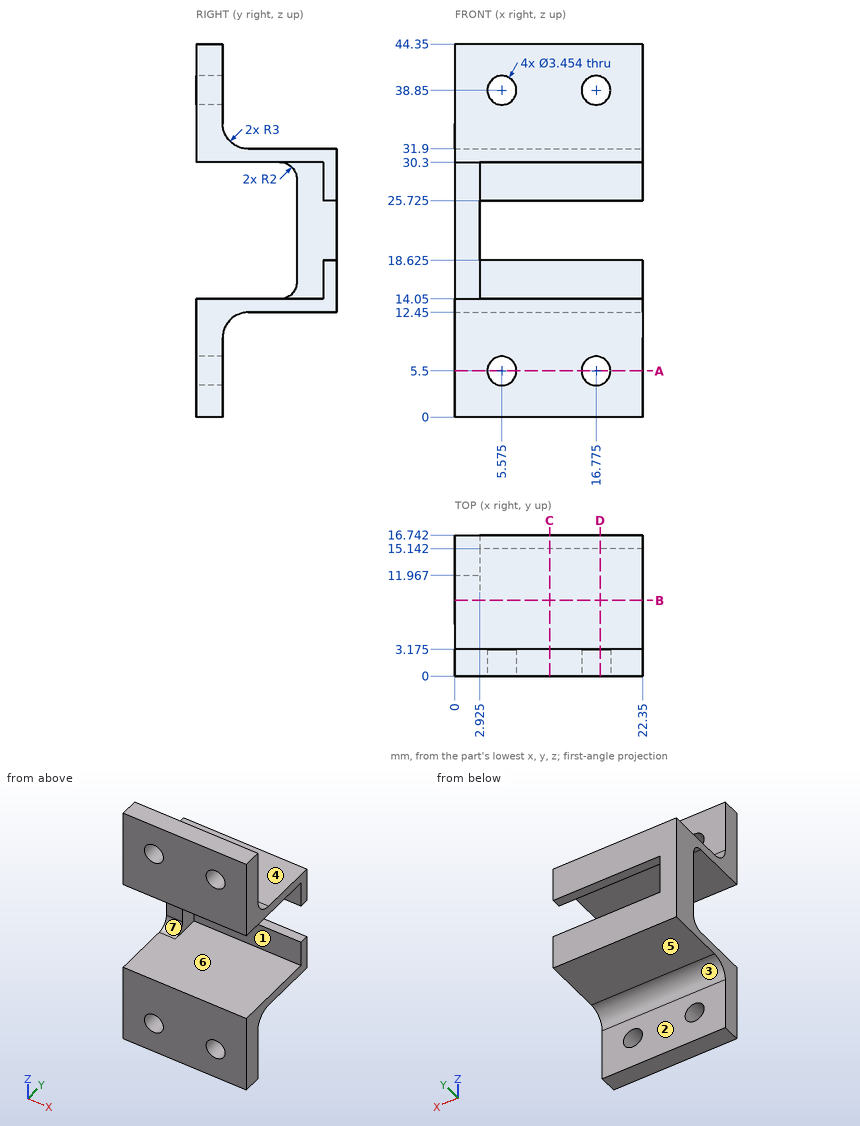
Part print with two shaded views. Sizes in mm from the minimum x, y, z corner. A direction names the side the tool comes from. Give positions to 0.01 mm unless a question says otherwise; leave off trailing zeros. Order: outer loops, then holes, each group sorted by start corner. A loop starts at its lowest first (then second) coordinate and runs counter-clockwise, first axis right, second up.
(1) Saw through at B-B, the plane y = 9. Give the cut face in (x, z), then the cut area to 3 significant figures.
(2) Saw through at C-C, the plane x = 11.25. Give the cut face in (y, z) (3 decimals), then the cut area to 3 significant figures.
(3) Saw through at D-D, the plane x = 17.25. Give the cut face in (y, z) (3 decimals).
(4) Tool access for the marked faces 5, 6 and 7: list every direction of +Z, -Z, +X, -X, +Y, -Y with a clear straight run to the whole face (end or side of a thin tool).
(5) Mould opens along Z. For the marked faces 1, 2, 3 and 4 say: released by +Z, released by -Z, zero draft, split by the parting line, or undercut.
(6) Saw through at A-A, the plane z = 5.5. Give the cut face in (x, y) (3 decimals).
(7) Drill centre lines: L1, parallel to X at y = 1.8, z = 5.5; L2, parallel to Z at x = 14, y = 14; L3, parallel to Z at x = 7.75, y = 2. Where is each one in solid material? Low to high.
(8) Flat gauge pins, fed straight in: pin 1 (8.5 mm diameter, centred on x = 15.5, y = 13, fed in from +Z); pin 2 (0.8 mm diameter, centred on x = 15.5, y = 16, fed in from -Z); pin 3 (5.5 mm diameter, centred on x = 5.575, z = 5.5, fed in from +Y) (3 decimals). Where does each tip first touch, or does it go through?
Results found:
1. outline: (0, 12.45) - (22.35, 12.45) - (22.35, 14.05) - (0, 14.05) - close; (0, 30.3) - (22.35, 30.3) - (22.35, 31.9) - (0, 31.9) - close
1. area: 71.5 mm2
2. outline: (0, 0) - (3.175, 0) - (3.175, 9.45) arc R3 cw to (6.175, 12.45) - (16.742, 12.45) - (16.742, 18.625) - (15.142, 18.625) - (15.142, 14.05) - (0, 14.05) - close; (0, 30.3) - (15.142, 30.3) - (15.142, 25.725) - (16.742, 25.725) - (16.742, 31.9) - (6.175, 31.9) arc R3 cw to (3.175, 34.9) - (3.175, 44.35) - (0, 44.35) - close
2. area: 151 mm2
3. outline: (0, 0) - (3.175, 0) - (3.175, 3.84) - (0, 3.84) - close; (0, 7.16) - (3.175, 7.16) - (3.175, 9.45) arc R3 cw to (6.175, 12.45) - (16.742, 12.45) - (16.742, 18.625) - (15.142, 18.625) - (15.142, 14.05) - (0, 14.05) - close; (0, 30.3) - (15.142, 30.3) - (15.142, 25.725) - (16.742, 25.725) - (16.742, 31.9) - (6.175, 31.9) arc R3 cw to (3.175, 34.9) - (3.175, 37.19) - (0, 37.19) - close; (0, 40.51) - (3.175, 40.51) - (3.175, 44.35) - (0, 44.35) - close
4. face 5: -Z, +X, -X, +Y
4. face 6: +X, -Y
4. face 7: +X, -X, -Y
5. face 1: undercut
5. face 2: zero draft
5. face 3: released by -Z
5. face 4: released by +Z
6. outline: (0, 0) - (3.848, 0) - (3.848, 3.175) - (0, 3.175) - close; (7.302, 0) - (15.048, 0) - (15.048, 3.175) - (7.302, 3.175) - close; (18.502, 0) - (22.35, 0) - (22.35, 3.175) - (18.502, 3.175) - close
7. L1: x = 0 to 3.85, 7.3 to 15.05, 18.5 to 22.35
7. L2: z = 12.45 to 14.05, 30.3 to 31.9
7. L3: z = 0 to 14.05, 30.3 to 44.35
8. pin 1: stops at z = 31.9
8. pin 2: stops at z = 12.45
8. pin 3: stops at y = 3.175
